from build123d import *

# Parameters (mm, degrees)
SKETCH1_W           = 20
SKETCH1_H           = 20
BOSS_EXTRUDE1_DEPTH = 1100
FILLET1_R           = 2
SKETCH2_W           = 16
SKETCH2_H           = 16
CUT_EXTRUDE1_DEPTH  = 1101
CUT_EXTRUDE2_DEPTH  = 21


with BuildPart() as part:
    # Sketch1 → Boss-Extrude1 (new body)
    with BuildSketch(Plane.XY):
        with Locations((279.9, -40.85)):
            Rectangle(SKETCH1_W, SKETCH1_H)
    extrude(amount=BOSS_EXTRUDE1_DEPTH)

    # Fillet1
    fillet1_edges = [part.edges().sort_by_distance(p)[0] for p in [
        (269.9, -30.85, 550),
        (289.9, -30.85, 550),
        (289.9, -50.85, 550),
        (269.9, -50.85, 550),
    ]]
    fillet(fillet1_edges, radius=FILLET1_R)

    # Sketch2 → Cut-Extrude1 (cut, through all)
    with BuildSketch(Plane.XY.offset(1100)):
        with Locations((279.9, -40.85)):
            Rectangle(SKETCH2_W, SKETCH2_H)
    extrude(amount=-CUT_EXTRUDE1_DEPTH, mode=Mode.SUBTRACT)

    # Sketch3 → Cut-Extrude2 (cut, through all)
    with BuildSketch(Plane.XZ.offset(50.85)):
        Polygon((269.9, 1100), (289.9, 1080), (289.9, 1100), align=None)
    extrude(amount=-CUT_EXTRUDE2_DEPTH, mode=Mode.SUBTRACT)


solid = part.part
The model under review builds one solid part; all positions refer to its coordinate system, in mm. Give positions to 0.01 mm unless a question says otherwise; leave off trailing zeros. Write each loop counter-clockwise with the first axis right and the second up, starting at its lowest first coordinate (ties: lowest second). Pieces come first, ordered by that corner, then holes. Notation, with made-up numbers: M -30.75,63.25 L -19.75,63.25 A19 ccw -19.75,73.25 Z; hole C 0.5,13 d9. An arc over 180 degrees is marked long. One line per question, with ' | ' between items. Start each with the question number.
Item 1: Wall thickness on line 1 (X direction, y = -36.25, z = 229.5); line 2 (Y direction, x = 285.5, z = 961); line 3 (X direction, y = -49.5, z = 178): over which ranges is each line inside the solid? List them lowest first. Write a range as from..to.
Item 2: We need section B-B on z = 183.5. Write out the cut boundary in (x, y).
Item 3: We need section A-A on x = 282.75. Write out the cut boundary in (y, z), plus the area to 3 significant figures.
Item 4: We need section C-C on y = -38.25. Write out the cut boundary in (x, z), plus the area to 3 significant figures.
Results found:
1) line 1: x = 269.9..271.9, 287.9..289.9 | line 2: y = -50.85..-48.85, -32.85..-30.85 | line 3: x = 270.01..289.79
2) outline: M 269.9,-48.85 A2 ccw 271.9,-50.85 L 287.9,-50.85 A2 ccw 289.9,-48.85 L 289.9,-32.85 A2 ccw 287.9,-30.85 L 271.9,-30.85 A2 ccw 269.9,-32.85 Z; hole M 271.9,-48.85 L 287.9,-48.85 L 287.9,-32.85 L 271.9,-32.85 Z
3) outline: M -50.85,0 L -48.85,0 L -48.85,1087.15 L -50.85,1087.15 Z; M -32.85,0 L -30.85,0 L -30.85,1087.15 L -32.85,1087.15 Z | area: 4,350 mm2
4) outline: M 269.9,0 L 271.9,0 L 271.9,1098 L 269.9,1100 Z; M 287.9,0 L 289.9,0 L 289.9,1080 L 287.9,1082 Z | area: 4,360 mm2
